```python
from build123d import *
from build123d.topology import SkipClean

# Parameters (mm, degrees)
BOSS_EXTRU_1_DEPTH      = 1.524
CONG_1_R                = 4.318
BOSS_EXTRU_3_START      = -1.524
BOSS_EXTRU_3_DEPTH      = 1.524
ESQUISSE3_R             = 1.8415
ENL_V_MAT_EXTRU_1_DEPTH = 127.347243097


with BuildPart() as part:
    # Esquisse1 → Boss.-Extru.1 (new body)
    with BuildSketch(Plane(origin=(0, 0, 0), x_dir=(1, 0, 0), z_dir=(0, 1, 0))):
        with BuildLine():
            Line((-95.25, 0), (95.25, 0))
            ThreePointArc((95.25, 0), (0, 83.82), (-95.25, 0))
        make_face()
    extrude(amount=BOSS_EXTRU_1_DEPTH)

    # Congé1
    cong_1_edges = [part.edges().sort_by_distance(p)[0] for p in [
        (-95.25, 0.762, 0),
        (95.25, 0.762, 0),
    ]]
    fillet(cong_1_edges, radius=CONG_1_R)

    # Esquisse2 → Boss.-Extru.3 (add)
    with BuildSketch(Plane(origin=(0, 1.524, 0), x_dir=(1, 0, 0), z_dir=(0, 1, 0)).offset(BOSS_EXTRU_3_START)):
        with BuildLine():
            ThreePointArc((61.910418509, 61.198651621), (61.671752387, 69.100962488), (53.997726446, 67.200224627))
            ThreePointArc((53.997726446, 67.200224627), (55.392549752, 66.233625302), (56.770074378, 65.24252883))
            ThreePointArc((56.770074378, 65.24252883), (59.71468664, 66.520695851), (59.277757535, 63.340515783))
            ThreePointArc((59.277757535, 63.340515783), (60.60355104, 62.281215121), (61.910418509, 61.198651621))
        make_face()
        with BuildLine():
            ThreePointArc((-53.997726446, 67.200224627), (-61.671752387, 69.100962488), (-61.910418509, 61.198651621))
            ThreePointArc((-61.910418509, 61.198651621), (-58.031708887, 64.301796789), (-53.997726446, 67.200224627))
        make_face()
    extrude(amount=BOSS_EXTRU_3_DEPTH)

    # Esquisse3 → Enlèv. mat.-Extru.1 (cut, through all)
    with SkipClean():  # the faces are left unmerged after this step: merging them gives an invalid solid
        with BuildSketch(Plane(origin=(0, 1.524, 0), x_dir=(1, 0, 0), z_dir=(0, 1, 0))):
            with Locations(Location((58.601845334, 65.053485411, 0), (0, 0, 270))):
                Circle(ESQUISSE3_R)
            with Locations(Location((-58.601845334, 65.053485411, 0), (0, 0, 270))):
                Circle(ESQUISSE3_R)
            with Locations(Location((58.601845334, 4.445, 0), (0, 0, 270))):
                Circle(ESQUISSE3_R)
            with Locations(Location((-58.601845334, 4.445, 0), (0, 0, 270))):
                Circle(ESQUISSE3_R)
        extrude(amount=-ENL_V_MAT_EXTRU_1_DEPTH, mode=Mode.SUBTRACT)


solid = part.part
```
Verification items for the finished model (mm, model axes). Coordinates: 2 decimals unless noted, no trailing zeros. Order: outer loops, then holes, each group sorted by start corner. A loop starts at its lowest first (then second) coordinate and runs counter-clockwise, first axis right, second up. Notation, with made-up numbers: (10.5, 80) -> (65.5, 80) arc R19 ccw to (65.5, 110) -> close; hole circle Ø7 at (87.5, 41). An arc over 180 degrees is marked (long way). Answer as CSV lines item,"result". Start each with the question number.
1) Cross-section at A-A, the plane y = 0.3. Record the boundary of the cut face in (x, z) (1 decimal).
2) Gauge pin test, flat end, axial feed: pin 1 Ø2 at (x, z) = (58.6, -4.44) entering from +Y. Record the tip position at first contact, or that the pin passes through.
3) Cross-section at B-B, the plane x = 81. Record the boundary of the cut face in (y, z), then the cut area to 3 significant figures.
4) Cross-section at C-C, the plane z = -25. Record the boundary of the cut face in (x, y).
5) Release check for a two-part mould opening along X. For faces 1 (the face through (-60.4, 0.77, -4.84)), 2 (the face through (-1, 0, -33)), 3 (the face through (83.295, 0.751, -35.577)), 4 (the face through (-59.307, 0.773, -63.352)) record: released by +X, released by -X, zero draft, split by the parting line, or undercut.
6) Material ranges on L1, parallel to Z at x = -60, y = 1.05; L2, parallel to X at y = 0.9, z = -5; L3, parallel to X at y = 1, z = -68.5, recorded low to high. Write a range as [from, to].
Conclusion:
1,outline,"(-94.5, -5.1) arc R96 ccw to (-61.9, -61.2) arc R5.1 ccw (long way) to (-54, -67.2) arc R96 ccw to (54, -67.2) arc R5.1 ccw (long way) to (61.9, -61.2) arc R96 ccw to (94.5, -5.1) arc R4.3 ccw to (90.2, 0) -> (-90.2, 0) arc R4.3 ccw to start; hole circle Ø3.7 at (-58.6, -65.1); hole circle Ø3.7 at (-58.6, -4.4); hole circle Ø3.7 at (58.6, -65.1); hole circle Ø3.7 at (58.6, -4.4)"
2,pin 1,"passes through"
3,outline,"(0, -39.37) -> (1.52, -39.37) -> (1.52, 0) -> (0, 0) -> close"
3,area,"60.0 mm²"
4,outline,"(-88.53, 0) -> (88.53, 0) -> (88.53, 1.52) -> (-88.53, 1.52) -> close"
5,face 1,"undercut"
5,face 2,"zero draft"
5,face 3,"released by +X"
5,face 4,"undercut"
6,L1,"z = [-69.94, -66.25], [-63.86, -5.64], [-3.25, 0]"
6,L2,"x = [-94.47, -60.36], [-56.85, 56.85], [60.36, 94.47]"
6,L3,"x = [-62.33, -54.87], [-52.03, 52.03], [54.87, 62.33]"
